Input: part model. Units: mm. Frame: model coordinates. Face numbers are marked on the shaded views. Coordinates: 2 decimals unless noted, no trailing zeros.
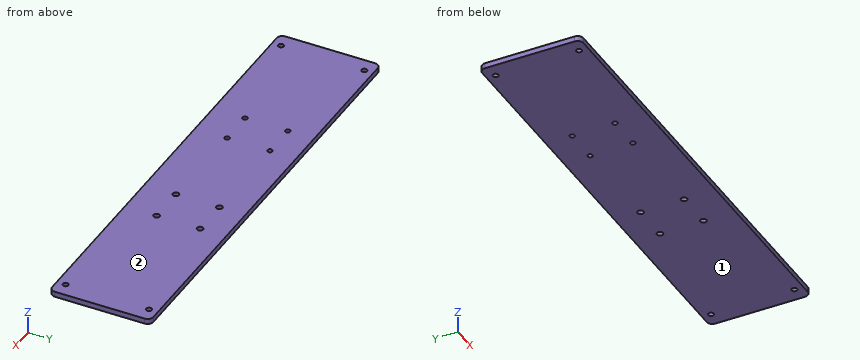
from build123d import *

# Parameters (mm, degrees)
SKETCH1_R           = 2.1
SKETCH1_R_2         = 1.9
SKETCH1_R_3         = 1.73
BOSS_EXTRUDE1_DEPTH = 3.8


with BuildPart() as part:
    # Sketch1 → Boss-Extrude1 (new body)
    with BuildSketch(Plane.XY):
        with BuildLine():
            Line((-10, -150.468857407), (-10, -87.916121505))
            ThreePointArc((-10, -87.916121505), (-8.828427125, -85.08769438), (-6, -83.916121505))
            Line((-6, -83.916121505), (296, -83.916121505))
            ThreePointArc((296, -83.916121505), (298.828427125, -85.08769438), (300, -87.916121505))
            Line((300, -87.916121505), (300, -150.468857407))
            ThreePointArc((300, -150.468857407), (298.828427125, -153.297284532), (296, -154.468857407))
            Line((296, -154.468857407), (-6, -154.468857407))
            ThreePointArc((-6, -154.468857407), (-8.828427125, -153.297284532), (-10, -150.468857407))
        make_face()
        with Locations(Location((172.212346295, -102, 0), (0, 0, 180))):
            Circle(SKETCH1_R, mode=Mode.SUBTRACT)
        with Locations(Location((290.004037955, -90.075164194, 0), (0, 0, 180))):
            Circle(SKETCH1_R_2, mode=Mode.SUBTRACT)
        with Locations(Location((290.004037955, -148.309814719, 0), (0, 0, 180))):
            Circle(SKETCH1_R_2, mode=Mode.SUBTRACT)
        with Locations(Location((-0.004037955, -148.309814719, 0), (0, 0, 180))):
            Circle(SKETCH1_R_2, mode=Mode.SUBTRACT)
        with Locations(Location((-0.004037955, -90.075164194, 0), (0, 0, 180))):
            Circle(SKETCH1_R_2, mode=Mode.SUBTRACT)
        with Locations(Location((198.212346295, -102, 0), (0, 0, 180))):
            Circle(SKETCH1_R, mode=Mode.SUBTRACT)
        with Locations(Location((172.212346295, -132.35, 0), (0, 0, 180))):
            Circle(SKETCH1_R, mode=Mode.SUBTRACT)
        with Locations(Location((198.212346295, -132.35, 0), (0, 0, 180))):
            Circle(SKETCH1_R, mode=Mode.SUBTRACT)
        with Locations(Location((79.683867595, -132.12, 0), (0, 0, 180))):
            Circle(SKETCH1_R_3, mode=Mode.SUBTRACT)
        with Locations(Location((79.683867595, -102.23, 0), (0, 0, 180))):
            Circle(SKETCH1_R_3, mode=Mode.SUBTRACT)
        with Locations(Location((103.743867595, -102.23, 0), (0, 0, 180))):
            Circle(SKETCH1_R_3, mode=Mode.SUBTRACT)
        with Locations(Location((103.743867595, -132.12, 0), (0, 0, 180))):
            Circle(SKETCH1_R_3, mode=Mode.SUBTRACT)
    extrude(amount=BOSS_EXTRUDE1_DEPTH)


solid = part.part
Item 1: Pin query (flat end, axial travel): pin 1 Ø6 at (x, y) = (0, -90.08) entering from +Z. Return the tip coordinate at first contact, or that it passes through.
Response values:
pin 1: stops at z = 3.8
Item 2: Draft query along Z for the marked faces 1 and 2. Return one class per face: pulls with the +Z half, pulls with the -Z half, needs draft (parallel to the pull), parting line crosses it, or undercut.
Response values:
face 1: pulls with the -Z half
face 2: pulls with the +Z half
Item 3: Ray query, probe 1 along X at (y, z) = (-102, 2.4); probe 2 along X at (y, z) = (-102.5, 0.7); probe 3 along X at (y, z) = (-134, 2.1). Return the intervals inside material, ascending.
Response values:
probe 1: x = -10 to 77.97, 81.4 to 102.03, 105.46 to 170.11, 174.31 to 196.11, 200.31 to 300
probe 2: x = -10 to 77.98, 81.39 to 102.04, 105.45 to 170.17, 174.25 to 196.17, 200.25 to 300
probe 3: x = -10 to 170.91, 173.51 to 196.91, 199.51 to 300
